```python
from build123d import *

# Parameters (mm, degrees)
F0_W     = 380
F0_H     = 380
F1_DEPTH = 350
F2_W     = 361
F2_H     = 331
F3_DEPTH = 361
F4_W     = 50.3650778532
F4_H     = 58.1228607893
F4_H_2   = 57.9308593273
F4_W_2   = 55.3338849545
F4_H_3   = 64.9694228172
F4_W_3   = 51.270159483
F5_DEPTH = 150
F6_W     = 444.3413615227
F6_H     = 444.3413615227
F6_W_2   = 380
F6_H_2   = 380
F7_DEPTH = 25


with BuildPart() as f1:
    # F0 (on Top) → F1 (new body)
    with BuildSketch(Plane.XY):
        Rectangle(F0_W, F0_H)
    extrude(amount=F1_DEPTH)

    # F2 (on face) → F3 (cut)
    with BuildSketch(Plane.XZ.offset(190)):
        with Locations((0, 175)):
            Rectangle(F2_W, F2_H)
    extrude(amount=-F3_DEPTH, mode=Mode.SUBTRACT)

    # F4 (on face) → F5 (join)
    with BuildSketch(Plane(origin=(0, 0, 0), x_dir=(1, 0, 0), z_dir=(0, 0, -1))):
        with Locations((164.8174610734, 160.9385696054)):
            Rectangle(F4_W, F4_H)
        with Locations((164.8174610734, -161.0345703363)):
            Rectangle(F4_W, F4_H_2)
        with Locations((-162.3330575228, -157.5152885914)):
            Rectangle(F4_W_2, F4_H_3)
        with Locations((-164.3649202585, 160.9385696054)):
            Rectangle(F4_W_3, F4_H)
    extrude(amount=F5_DEPTH)

    # F6 (on face) → F7 (join)
    with BuildSketch(Plane.XY.offset(350)):
        Rectangle(F6_W, F6_H)
        Rectangle(F6_W_2, F6_H_2, mode=Mode.SUBTRACT)
        Rectangle(F6_W_2, F6_H_2)
    extrude(amount=F7_DEPTH)


solid = f1.part
```
For this review, take the finished solid that the model builds, in its own axes (mm). A direction names the side the tool comes from. Coordinates: 2 decimals unless noted, no trailing zeros. Loops run counter-clockwise (first coordinate to the right, second up) from the corner with the lowest first, then second, coordinate; pieces in that order, holes last.
1. Add section A-A, the plane y = -110.5. Give the boundary of the cut face in (x, z), then the cut area to 3 significant figures.
2. Add section D-D, the plane z = 276.5. Give the boundary of the cut face in (x, y).
3. For faces 1 (the flat face through (164, -131.877, -74)), 2 (the flat face through (-3, -12, 340.5)), 3 (the flat face through (190, 3, 159)), 4 (the flat face through (-134.666, 158, -74)), 5 (the flat face through (-29, -190, 9)), list the 3-axis set-ups (+Z, -Z, +X, -X, +Y, -Y) from which the entire face can be reached by the end or side of a thin tool; tool diameter is ignored.
4. Mouldability with a two-part tool opening along Y and no side actions: class faces 6 (the flat face through (-165, -131.877, -74)), 7 (the flat face through (-165, -161, -150)), 8 (the flat face through (-3, 3, 0)), 9 (the flat face through (-3, 222.171, 362)) as +Y half, -Y half, draft (parallel to the pull), parting line (faces both ways), or undercut.
5. For line 1 (X direction, y = 19.5, z = 52); line 2 (Z direction, x = 122.5, y = -8); line 3 (Z direction, x = -160, y = 149), list the stretches that pass through material, from the lowest coordinate up.
6. Insertion check: P1, Ø1.5, axis at y = -138.5, z = -57.5, coming from the +X side; P2, Ø1.5, axis at x = -102, y = -15.5, coming from the -Z side; P3, Ø1.5, axis at x = 41.5, z = 181, coming from the -Y side. Each pin has a flat end and moves straight along its axis. Give the tip position at first contact, or say it passes through.
7. Add section C-C, the plane x = 61. Give the boundary of the cut face in (y, z).
8. Add section B-B, the plane z = -104.5. Give the boundary of the cut face in (x, y).
Result:
1. outline: (-222.17, 350) - (-190, 350) - (-190, 0) - (190, 0) - (190, 350) - (222.17, 350) - (222.17, 375) - (-222.17, 375) - close; hole (-180.5, 9.5) - (180.5, 9.5) - (180.5, 340.5) - (-180.5, 340.5) - close
1. area: 24,600 mm2
2. outline: (-190, -190) - (-180.5, -190) - (-180.5, 171) - (180.5, 171) - (180.5, -190) - (190, -190) - (190, 190) - (-190, 190) - close
3. face 1: -Z, +X, -X
3. face 2: -Y
3. face 3: -Z, +X, +Y, -Y
3. face 4: -Z, +Y, -Y
3. face 5: -Z, +X, -X, -Y
4. face 6: undercut
4. face 7: draft
4. face 8: undercut
4. face 9: +Y half
5. line 1: x = -190 to -180.5, 180.5 to 190
5. line 2: z = 0 to 9.5, 340.5 to 375
5. line 3: z = -150 to 9.5, 340.5 to 375
6. P1: stops at x = 190
6. P2: stops at z = 0
6. P3: stops at y = 171
7. outline: (-222.17, 350) - (-190, 350) - (-190, 340.5) - (171, 340.5) - (171, 9.5) - (-190, 9.5) - (-190, 0) - (190, 0) - (190, 350) - (222.17, 350) - (222.17, 375) - (-222.17, 375) - close
8. outline: (-190, -190) - (-138.73, -190) - (-138.73, -131.88) - (-190, -131.88) - close; (-190, 125.03) - (-134.67, 125.03) - (-134.67, 190) - (-190, 190) - close; (139.63, -190) - (190, -190) - (190, -131.88) - (139.63, -131.88) - close; (139.63, 132.07) - (190, 132.07) - (190, 190) - (139.63, 190) - close
